from build123d import *

# Parameters (mm, degrees)
SKETCH_1_R          = 2.75
SKETCH_1_R_2        = 2.5
EXTRUDE_1_DEPTH     = 4
CHAMFER_2_SIZE      = 2
SKETCH_2_R          = 1.025
CUT_EXTRUDE_1_DEPTH = 5


with BuildPart() as part:
    # 草图1 → 凸台-拉伸1 (new body)
    with BuildSketch(Plane(origin=(0, 0, 0), x_dir=(1, 0, 0), z_dir=(0, 1, 0))):
        with BuildLine():
            Line((38, -4.5), (18, -4.5))
            Line((18, -4.5), (18, -24.5))
            Line((18, -24.5), (33.644053232, -24.5))
            ThreePointArc((33.644053232, -24.5), (34.63190154, -25.344578889), (33.951118195, -26.451688557))
            Line((33.951118195, -26.451688557), (2.456519701, -36.613508453))
            ThreePointArc((2.456519701, -36.613508453), (-4.708919324, -35.467308467), (-8, -29))
            Line((-8, -29), (-8, 11.5))
            ThreePointArc((-8, 11.5), (-0.67766953, 29.17766953), (17, 36.5))
            Line((17, 36.5), (33, 36.5))
            ThreePointArc((33, 36.5), (36.535533906, 35.035533906), (38, 31.5))
            Line((38, 31.5), (38, -4.5))
        make_face()
        with Locations((28, 5.5)):
            Circle(SKETCH_1_R, mode=Mode.SUBTRACT)
        with Locations((28, 25.5)):
            Circle(SKETCH_1_R, mode=Mode.SUBTRACT)
        with Locations((0, 5.5)):
            Circle(SKETCH_1_R_2, mode=Mode.SUBTRACT)
        with Locations((0, -24.5)):
            Circle(SKETCH_1_R_2, mode=Mode.SUBTRACT)
    extrude(amount=EXTRUDE_1_DEPTH)

    # 倒角2
    chamfer_2_edges = [part.edges().sort_by_distance(p)[0] for p in [
        (25.25, 0, -25.5),
    ]]
    chamfer(chamfer_2_edges, length=CHAMFER_2_SIZE)

    # 草图2 → 切除-拉伸1 (cut, symmetric)
    with BuildSketch(Plane(origin=(0, 4, 0), x_dir=(1, 0, 0), z_dir=(0, 1, 0))):
        with Locations((18, -4.5)):
            Circle(SKETCH_2_R)
        with Locations((18, -24.5)):
            Circle(SKETCH_2_R)
    extrude(amount=CUT_EXTRUDE_1_DEPTH, both=True, mode=Mode.SUBTRACT)


solid = part.part
The listing builds one solid part. Answer for the finished solid, in the listing's coordinates (mm). A direction names the side the tool comes from. Coordinates: 2 decimals unless noted, no trailing zeros. Loops run counter-clockwise (first coordinate to the right, second up) from the corner with the lowest first, then second, coordinate; pieces in that order, holes last. Notation, with made-up numbers: (35.25, 40) -> (74.25, 40) arc R12 ccw to (74.25, 61) -> close; hole circle Ø3 at (-26.75, 41.5). An arc over 180 degrees is marked (long way). Answer in a Markdown table with one row per item. Add a question column.
1. The part is cut by section A-A, the plane z = -5.5. Write down the section's boundary in (x, y), then the cut area to 3 significant figures.
2. For faces 1 (the flat face through (26, 2, 24.5)), 2 (the cylindrical face through (0, 2, 22)), determine the directions among +Z, -Z, +X, -X, +Y, -Y from which every point of the face is accessible in a straight line to the end or side of a thin tool.
3. Flat-ended cylindrical pins translate along their axes: P1, Ø1.2, axis at x = 18, z = 24.5, coming from the -Y side; P2, Ø1.5, axis at x = 7, y = 1, coming from the +Z side; P3, Ø2, axis at y = 1.5, z = 18, coming from the +X side. Find the tip coordinate at first contact, or state that the pin passes through.
4. The part is cut by section B-B, the plane y = 0.65. Count the separate pieces of the cut face and the enclosed holes in it, then the cut area to 3 significant figures.
5. The part is cut by section C-C, the plane x = 0. Write down the section's boundary in (y, z), then the cut area to 3 significant figures.
6. Determine the mould class of faces 3 (the cylindrical face through (0, 2, -8)), 4 (the cylindrical face through (-4.62, 1.97, 35.53)), 5 (the flat face through (18, 2, 14)), 6 (the flat face through (38, 2, -14)) for opening direction Z: +Z half, -Z half, draft (parallel to the pull), parting line (faces both ways), or undercut.
7. The part is cut by section D-D, the plane z = 21. Write down the section's boundary in (x, y).
8. Consider line 1 (X direction, y = 3.2, z = -5.5); line 2 (Z direction, x = 28, y = 3.5); line 3 (X direction, y = 3, z = -6). Determine where each line is inside the solid, lowest interval first. Write a range as [from, to].
Answer below:
| question | item | result |
|---|---|---|
| 1 | outline | (-8, 0) -> (-2.5, 0) -> (-2.5, 4) -> (-8, 4) -> close; (2.5, 0) -> (25.25, 0) -> (25.25, 4) -> (2.5, 4) -> close; (30.75, 0) -> (38, 0) -> (38, 4) -> (30.75, 4) -> close |
| 1 | area | 142 mm2 |
| 2 | face 1 | +X, +Y, -Y |
| 2 | face 2 | +Y, -Y |
| 3 | P1 | through |
| 3 | P2 | z = 35.39 |
| 3 | P3 | x = 18 |
| 4 | separate pieces | 1 |
| 4 | enclosed holes | 4 |
| 4 | area | 2,480 mm2 |
| 5 | outline | (0, -29.83) -> (4, -29.83) -> (4, -8) -> (0, -8) -> close; (0, -3) -> (4, -3) -> (4, 22) -> (0, 22) -> close; (0, 27) -> (4, 27) -> (4, 37) -> (0, 37) -> close |
| 5 | area | 227 mm2 |
| 6 | face 3 | undercut |
| 6 | face 4 | +Z half |
| 6 | face 5 | undercut |
| 6 | face 6 | draft |
| 7 | outline | (-8, 0) -> (18, 0) -> (18, 4) -> (-8, 4) -> close |
| 8 | line 1 | [-8, -2.5], [2.5, 25.25], [30.75, 38] |
| 8 | line 2 | [-36.5, -28.25], [-22.75, -8.25], [-2.75, 4.5], [24.5, 28.37] |
| 8 | line 3 | [-8, -2.45], [2.45, 25.3], [30.7, 38] |
